Geometry check sheet. Reference: the model listing, model coordinates, mm. Face numbers are marked on the shaded views. Round coordinates to 2 decimals unless told otherwise and drop trailing zeros. Order: outer loops, then holes, each group sorted by start corner. A loop starts at its lowest first (then second) coordinate and runs counter-clockwise, first axis right, second up.
(1) Sectioned sample at B-B (y = -3). Record the boundary of the cut face in (x, z), plus the area to 3 significant figures.
(2) Sectioned sample at A-A (x = -4.5). Record the boundary of the cut face in (y, z).
(3) Sectioned sample at C-C (x = -12.2). Record the boundary of the cut face in (y, z), plus the area to 3 significant figures.
(4) Go/stop test with a flat-tipped pin: pin 1 (4 mm diameter, centred on y = -6.5, z = 2.5, fed in from -X). Record where the tip stops, or that it passes through.
(5) Release check for a two-part mould opening along X. For the marked faces 1 and 2 record: +X half, -X half, draft (parallel to the pull), parting line (faces both ways), or undercut.
(6) Material ranges on line 1 along Z through (x, y) = (4.5, -7.5); line 2 along Z through (x, y) = (-12.2, -1.75); line 3 along X through (y, z) = (-5, 1.5), recorded low to high.
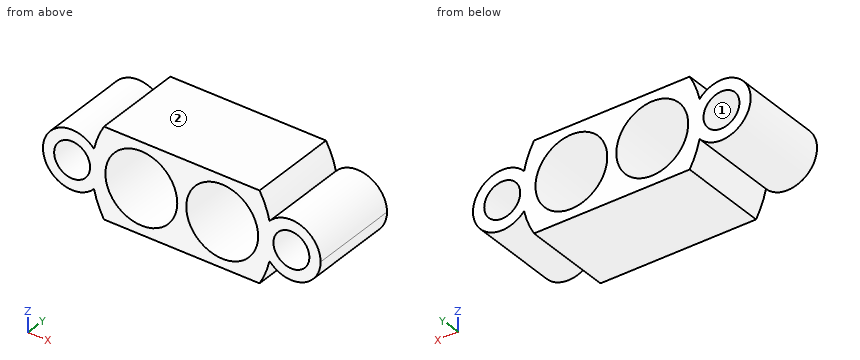
from build123d import *

# Parameters (mm, degrees)
F0_R     = 4
F1_DEPTH = 10
F0_R_2   = 2
F2_DEPTH = 10
F3_DEPTH = 10


with BuildPart() as f1:
    # F0 (on Front) → F1 (new body)
    with BuildSketch(Plane.XZ):
        with BuildLine():
            ThreePointArc((9.7654713115, -2.1530374044), (8.95, 0), (9.7654713115, 2.1530374044))
            ThreePointArc((9.7654713115, 2.1530374044), (9.322185241, 3.618958736), (8.6602540378, 5))
            Line((8.6602540378, 5), (-8.6602540378, 5))
            ThreePointArc((-8.6602540378, 5), (-9.322185241, 3.618958736), (-9.7654713115, 2.1530374044))
            ThreePointArc((-9.7654713115, 2.1530374044), (-9.1606975934, 1.1511476366), (-8.95, 0))
            ThreePointArc((-8.95, 0), (-9.1606975934, -1.1511476366), (-9.7654713115, -2.1530374044))
            ThreePointArc((-9.7654713115, -2.1530374044), (-9.322185241, -3.618958736), (-8.6602540378, -5))
            Line((-8.6602540378, -5), (8.6602540378, -5))
            ThreePointArc((8.6602540378, -5), (9.322185241, -3.618958736), (9.7654713115, -2.1530374044))
        make_face()
        with Locations((-4.5, 0)):
            Circle(F0_R, mode=Mode.SUBTRACT)
        with Locations((4.5, 0)):
            Circle(F0_R, mode=Mode.SUBTRACT)
    extrude(amount=F1_DEPTH)

    # F0 (on Front) → F2 (join)
    with BuildSketch(Plane.XZ):
        with BuildLine():
            ThreePointArc((-9.7654713115, -2.1530374044), (-10, 0), (-9.7654713115, 2.1530374044))
            ThreePointArc((-9.7654713115, 2.1530374044), (-15.45, 0), (-9.7654713115, -2.1530374044))
        make_face()
        with Locations((-12.2, 0)):
            Circle(F0_R_2, mode=Mode.SUBTRACT)
        with BuildLine():
            ThreePointArc((9.7654713115, 2.1530374044), (9.941194926, 1.082886625), (10, 0))
            ThreePointArc((10, 0), (9.941194926, -1.082886625), (9.7654713115, -2.1530374044))
            ThreePointArc((9.7654713115, -2.1530374044), (13.3511476366, -3.0393024066), (15.45, 0))
            ThreePointArc((15.45, 0), (13.3511476366, 3.0393024066), (9.7654713115, 2.1530374044))
        make_face()
        with Locations((12.2, 0)):
            Circle(F0_R_2, mode=Mode.SUBTRACT)
    extrude(amount=F2_DEPTH)

    # F0 (on Front) → F3 (join)
    with BuildSketch(Plane.XZ):
        with BuildLine():
            ThreePointArc((9.7654713115, -2.1530374044), (9.941194926, -1.082886625), (10, 0))
            ThreePointArc((10, 0), (9.941194926, 1.082886625), (9.7654713115, 2.1530374044))
            ThreePointArc((9.7654713115, 2.1530374044), (8.95, 0), (9.7654713115, -2.1530374044))
        make_face()
        with BuildLine():
            ThreePointArc((-8.95, 0), (-9.1606975934, 1.1511476366), (-9.7654713115, 2.1530374044))
            ThreePointArc((-9.7654713115, 2.1530374044), (-10, 0), (-9.7654713115, -2.1530374044))
            ThreePointArc((-9.7654713115, -2.1530374044), (-9.1606975934, -1.1511476366), (-8.95, 0))
        make_face()
    extrude(amount=F3_DEPTH)


solid = f1.part
Answer below:
1. outline: (-9.77, -2.15) arc R10 ccw to (-8.66, -5) - (8.66, -5) arc R10 ccw to (9.77, -2.15) arc R3.25 ccw (long way) to (9.77, 2.15) arc R10 ccw to (8.66, 5) - (-8.66, 5) arc R10 ccw to (-9.77, 2.15) arc R3.25 ccw (long way) to start; hole circle Ø4 at (-12.2, 0); hole circle Ø8 at (-4.5, 0); hole circle Ø8 at (4.5, 0); hole circle Ø4 at (12.2, 0)
1. area: 126 mm2
2. outline: (-10, -5) - (0, -5) - (0, -4) - (-10, -4) - close; (-10, 4) - (0, 4) - (0, 5) - (-10, 5) - close
3. outline: (-10, -3.25) - (0, -3.25) - (0, -2) - (-10, -2) - close; (-10, 2) - (0, 2) - (0, 3.25) - (-10, 3.25) - close
3. area: 25.0 mm2
4. pin 1: stops at x = -15.41
5. face 1: undercut
5. face 2: draft
6. line 1: z = -5 to -4, 4 to 5
6. line 2: z = -3.25 to -2, 2 to 3.25
6. line 3: x = -15.08 to -13.52, -10.88 to -8.21, -0.79 to 0.79, 8.21 to 10.88, 13.52 to 15.08
